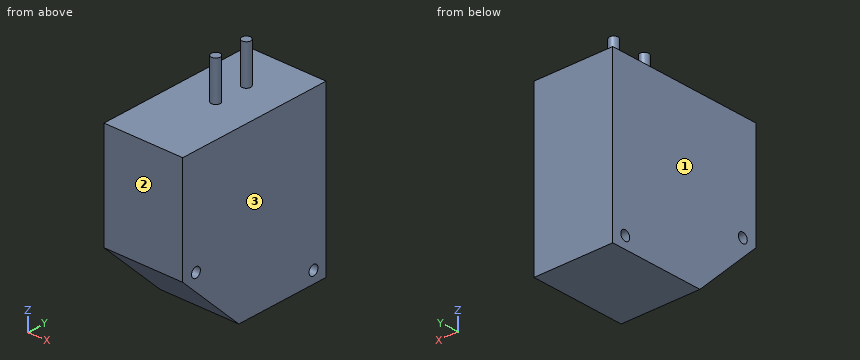
```python
from build123d import *

# Parameters (mm, degrees)
BOSS_EXTRUDE1_DEPTH        = 20
F_2_5_2_5_DIAMETER_HOLE1_D = 2.5
F_2_5_2_5_DIAMETER_HOLE2_D = 2.5
SKETCH6_R                  = 1.125
BOSS_EXTRUDE2_DEPTH        = 10


with BuildPart() as part:
    # Sketch1 → Boss-Extrude1 (new body)
    with BuildSketch(Plane(origin=(0, 0, 0), x_dir=(0, 0, -1), z_dir=(1, 0, 0))):
        Polygon((5.7, -20.05), (21.1, -4.35), (21.1, 20.05), (-21.1, 20.05), (-21.1, -20.05), align=None)
    extrude(amount=BOSS_EXTRUDE1_DEPTH)

    # Ø2.5 (2.5) Diameter Hole1 (through all)
    with Locations(Plane(origin=(20, 0, 0), x_dir=(0, 0, -1), z_dir=(1, 0, 0))):
        with Locations((18.1, 16.55)):
            Hole(F_2_5_2_5_DIAMETER_HOLE1_D / 2)

    # Ø2.5 (2.5) Diameter Hole2 (through all)
    with Locations(Plane(origin=(20, 0, 0), x_dir=(0, 0, -1), z_dir=(1, 0, 0))):
        with Locations((5.1, -16.35)):
            Hole(F_2_5_2_5_DIAMETER_HOLE2_D / 2)

    # Sketch6 → Boss-Extrude2 (add)
    with BuildSketch(Plane.XY.offset(21.1)):
        with Locations(Location((10, 8.75, 0), (0, 0, 90))):
            Circle(SKETCH6_R)
        with Locations(Location((10, 0.2, 0), (0, 0, 90))):
            Circle(SKETCH6_R)
    extrude(amount=BOSS_EXTRUDE2_DEPTH)


solid = part.part
```
Can you work these out from the model? Positions are in its coordinate system, mm. Face numbers are marked on the shaded views. Coordinates: 2 decimals unless noted, no trailing zeros. Loops run counter-clockwise (first coordinate to the right, second up) from the corner with the lowest first, then second, coordinate; pieces in that order, holes last. Notation, with made-up numbers: (-13.75, 45) -> (38.25, 45) arc R24 cw to (38.25, 68) -> close; hole circle Ø11 at (-6.75, -23). An arc over 180 degrees is marked (long way). Put each result on its own line as item: value. Start each with the question number.
Q1. I want a section at B-B (y = 8.75). Write out the boundary of the cut face in (x, z) (3 decimals), plus the area to 4 significant figures.
Q2. I want a section at A-A (z = -5.1). Write out the boundary of the cut face in (x, y).
Q3. Thinking about a two-plate mould opening in X: for the marked faces 1, 2 and 3, which applies, pulls with the +X half, pulls with the -X half, needs draft (parallel to the pull), parting line crosses it, or undercut?
Q4. I want a section at D-D (y = -16.35). Write out the boundary of the cut face in (x, z), plus the area to 3 significant figures.
Q5. I'm going to push flat-ended pins straight in: P1, Ø1.5, axis at x = 2, y = 3, coming from the +Z side; P2, Ø10, axis at x = 8, y = -13, coming from the -Z side. Where does each tip first touch, or does it pass through?
Q6. I want a section at C-C (x = 14.75). Write out the boundary of the cut face in (y, z), plus the area to 3 significant figures.
Q7. If I drill on line 1 (Y direction, x = 13, z = -5.1); line 2 (Y direction, x = 12.75, z = -18.1); line 3 (Z direction, x = 11.75, y = 16), over which ranges is the centre line in solid material (lowest first)? Write a range as [from, to].
Taken from the geometry:
1. outline: (0, -21.1) -> (20, -21.1) -> (20, 21.1) -> (11.125, 21.1) -> (11.125, 31.1) -> (8.875, 31.1) -> (8.875, 21.1) -> (0, 21.1) -> close
1. area: 866.5 mm2
2. outline: (0, -20.05) -> (20, -20.05) -> (20, -17.6) -> (0, -17.6) -> close; (0, -15.1) -> (20, -15.1) -> (20, 20.05) -> (0, 20.05) -> close
3. face 1: pulls with the -X half
3. face 2: needs draft
3. face 3: pulls with the +X half
4. outline: (0, -9.33) -> (20, -9.33) -> (20, -6.35) -> (0, -6.35) -> close; (0, -3.85) -> (20, -3.85) -> (20, 21.1) -> (0, 21.1) -> close
4. area: 559 mm2
5. P1: stops at z = 21.1
5. P2: stops at z = -17.52
6. outline: (-20.05, -5.7) -> (-4.35, -21.1) -> (20.05, -21.1) -> (20.05, 21.1) -> (-20.05, 21.1) -> close; hole circle Ø2.5 at (-16.35, -5.1); hole circle Ø2.5 at (16.55, -18.1)
6. area: 1,560 mm2
7. line 1: y = [-20.05, -17.6], [-15.1, 20.05]
7. line 2: y = [-7.41, 15.3], [17.8, 20.05]
7. line 3: z = [-21.1, -19.22], [-16.98, 21.1]
